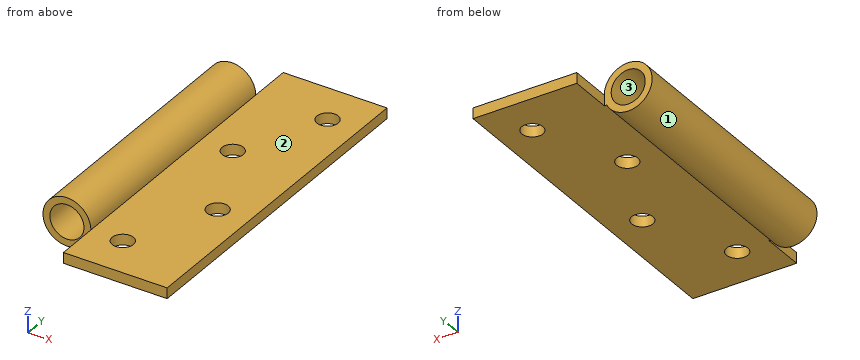
from build123d import *

# Parameters (mm, degrees)
F0_R     = 5.08
F1_DEPTH = 50.8
F2_W     = 14.402608
F2_H     = 12.7
F2_H_2   = 12.700002
F3_DEPTH = 12.7
F5_D     = 6.35


with BuildPart() as f1:
    # F0 (on Front) → F1 (new body, symmetric)
    with BuildSketch(Plane.XZ):
        with BuildLine():
            ThreePointArc((6.399417, 0), (6.955178, 1.544459), (7.14375, 3.175))
            ThreePointArc((7.14375, 3.175), (-6.955178, 4.805541), (6.399417, 0))
        make_face()
        with Locations((0, 3.175)):
            Circle(F0_R, mode=Mode.SUBTRACT)
        with BuildLine():
            Line((38.1, 3.175), (7.14375, 3.175))
            ThreePointArc((7.14375, 3.175), (6.955178, 1.544459), (6.399417, 0))
            Line((6.399417, 0), (38.1, 0))
            Line((38.1, 0), (38.1, 3.175))
        make_face()
    extrude(amount=F1_DEPTH, both=True)

    # F2 (on Top) → F3 (cut, symmetric)
    with BuildSketch(Plane.XY):
        with Locations((-0.057554, 44.45)):
            Rectangle(F2_W, F2_H)
        with Locations((-0.057554, -44.449999)):
            Rectangle(F2_W, F2_H_2)
    extrude(amount=F3_DEPTH, both=True, mode=Mode.SUBTRACT)

    # F5 (through all)
    with Locations(Plane.XY.offset(3.175)):
        with Locations((28.575, 38.1), (16.66875, 12.7), (28.575, -12.7), (16.66875, -38.1)):
            Hole(F5_D / 2)


solid = f1.part
Source: CAD feature listing. Evaluate the final solid. Frame: model axes, mm. Face numbers are marked on the shaded views. Round coordinates to 2 decimals unless told otherwise and drop trailing zeros. Loops run counter-clockwise (first coordinate to the right, second up) from the corner with the lowest first, then second, coordinate; pieces in that order, holes last. Notation, with made-up numbers: (-29, 3.25) - (22, 3.25) arc R30 cw to (22, 41.25) - close; hole circle Ø4 at (2, -34). An arc over 180 degrees is marked (long way). Write item = value, one per line. Start each with the question number.
Item 1: First-contact query: pin 1 Ø9.5 at (x, y) = (15, 6) entering from -Z; pin 2 Ø4 at (x, y) = (23.5, -4.5) entering from +Z (3 decimals); pin 3 Ø1.6 at (y, z) = (45, 1) entering from -X. Flat tips, straight axial feed; report the tip coordinate or a pass-through.
Item 2: Mould query, pull axis X, two halves, no side actions, for the marked faces 1, 2 and 3. Classes: released by +X, released by -X, zero draft, split by the parting line, or undercut.
Item 3: Material intervals for line 1 (Z direction, x = 0, y = -11) (3 decimals); line 2 (Z direction, x = 30, y = 9) (3 decimals); line 3 (X direction, y = 0, z = 4.5), sorted ascending.
Item 4: Section query B-B on x = 0. Output: boundary loops of the cut face in (y, z) (3 decimals), plus the area to 3 significant figures.
Item 5: Section query C-C on z = 6.25. Output: boundary loops of the cut face in (x, y).
Item 6: Section query A-A on y = 12.7. Output: boundary loops of the cut face in (x, z) (1 decimal).
Item 7: Section query D-D on y = -8. Output: boundary loops of the cut face in (x, z) (1 decimal), plus the area to 3 significant figures.
Results list:
q1.pin_1 = 0
q1.pin_2 = 3.175
q1.pin_3 = 7.14
q2.face_1 = split by the parting line
q2.face_2 = zero draft
q2.face_3 = undercut
q3.line_1 = -3.969 to -1.905, 8.255 to 10.319
q3.line_2 = 0 to 3.175
q3.line_3 = -7.02 to -4.9, 4.9 to 7.02
q4.outline = (-38.1, -3.969) - (38.1, -3.969) - (38.1, -1.905) - (-38.1, -1.905) - close; (-38.1, 8.255) - (38.1, 8.255) - (38.1, 10.319) - (-38.1, 10.319) - close
q4.area = 315 mm²
q5.outline = (-6.45, -38.1) - (-4.04, -38.1) - (-4.04, 38.1) - (-6.45, 38.1) - close; (4.04, -38.1) - (6.45, -38.1) - (6.45, 38.1) - (4.04, 38.1) - close
q6.outline = (6.4, 0) - (13.5, 0) - (13.5, 3.2) - (7.1, 3.2) arc R7.1 ccw (long way) to start; (19.8, 0) - (38.1, 0) - (38.1, 3.2) - (19.8, 3.2) - close; hole circle Ø10.2 at (0, 3.2)
q7.outline = (6.4, 0) - (38.1, 0) - (38.1, 3.2) - (7.1, 3.2) arc R7.1 ccw (long way) to start; hole circle Ø10.2 at (0, 3.2)
q7.area = 178 mm²
